from build123d import *

# Parameters (mm, degrees)
SKETCH1_W                      = 114.3
SKETCH1_H                      = 63.5
BASE_FLANGE1_DEPTH             = 2.032
EDGE_FLANGE1_STRIP_W           = 14.478
EDGE_FLANGE1_STRIP_H           = 2.032
EDGE_FLANGE1_STRIP_CUT_DEPTH   = 114.3
EDGE_FLANGE1_STRIP_2_W         = 14.478
EDGE_FLANGE1_STRIP_2_H         = 2.032
EDGE_FLANGE1_STRIP_CUT_2_DEPTH = 114.3
EDGE_FLANGE1_DEPTH             = 114.3
EDGE_FLANGE1_BEND_DEPTH        = 114.3
EDGE_FLANGE2_DEPTH             = 63.5
EDGE_FLANGE2_2_DEPTH           = 5.207
EDGE_FLANGE2_START             = 58.293
EDGE_FLANGE2_3_DEPTH           = 5.207
EDGE_FLANGE2_START_2           = 5.207
EDGE_FLANGE2_4_DEPTH           = 53.086
SKETCH15_R                     = 2.45745
CUT_EXTRUDE1_DEPTH             = 135.089147674
FILLET1_R                      = 3.175


# Read off the part's stored shape, not the designer's step: Edge-Flange2
# Sheet-metal steps are written as plain solids
with BuildPart() as part:
    # Sketch1 → Base-Flange1 (new body)
    with BuildSketch(Plane(origin=(0, 0, 0), x_dir=(0, 0, -1), z_dir=(1, 0, 0))):
        with Locations((57.15, 31.75)):
            Rectangle(SKETCH1_W, SKETCH1_H)
    extrude(amount=-BASE_FLANGE1_DEPTH)

    # Edge-Flange1 strip (across the edge) → Edge-Flange1 strip cut (cut)
    with BuildSketch(Plane(origin=(0, 63.5, -114.3), x_dir=(0, -1, 0), z_dir=(0, 0, 1))):
        with Locations((-2.032, -1.016)):
            Rectangle(EDGE_FLANGE1_STRIP_W, EDGE_FLANGE1_STRIP_H)
    extrude(amount=EDGE_FLANGE1_STRIP_CUT_DEPTH, mode=Mode.SUBTRACT)

    # Edge-Flange1 strip 2 (across the edge) → Edge-Flange1 strip cut 2 (cut)
    with BuildSketch(Plane.YX):
        with Locations((-2.032, -1.016)):
            Rectangle(EDGE_FLANGE1_STRIP_2_W, EDGE_FLANGE1_STRIP_2_H)
    extrude(amount=EDGE_FLANGE1_STRIP_CUT_2_DEPTH, mode=Mode.SUBTRACT)

    # Edge-Flange1 section (across the edge) → Edge-Flange1 (add)
    with BuildSketch(Plane(origin=(0, 63.5, -114.3), x_dir=(0, -1, 0), z_dir=(0, 0, 1))):
        with BuildLine():
            Line((0, 3.175), (0, 29.718))
            Line((0, 29.718), (2.032, 29.718))
            Line((2.032, 29.718), (2.032, 3.175))
            ThreePointArc((2.032, 3.175), (2.96193597, 0.92993597), (5.207, 0))
            Line((5.207, 0), (5.207, -2.032))
            ThreePointArc((5.207, -2.032), (1.52509499, -0.50690501), (0, 3.175))
        make_face()
    extrude(amount=EDGE_FLANGE1_DEPTH)

    # Edge-Flange1 section 2 (across the edge) → Edge-Flange1 bend (add)
    with BuildSketch(Plane.YX):
        with BuildLine():
            Line((0, 3.175), (0, 29.718))
            Line((0, 29.718), (2.032, 29.718))
            Line((2.032, 29.718), (2.032, 3.175))
            ThreePointArc((2.032, 3.175), (2.96193597, 0.92993597), (5.207, 0))
            Line((5.207, 0), (5.207, -2.032))
            ThreePointArc((5.207, -2.032), (1.52509499, -0.50690501), (0, 3.175))
        make_face()
    extrude(amount=EDGE_FLANGE1_BEND_DEPTH)

    # Edge-Flange2 outline → Edge-Flange2 (cut)
    with BuildSketch(Plane(origin=(0, 0, 0), x_dir=(1, 0, 0), z_dir=(0, 1, 0))):
        with BuildLine():
            Line((3.175, 0), (3.175, 3.175))
            Line((3.175, 3.175), (0, 3.175))
            ThreePointArc((0, 3.175), (0.92993597, 0.92993597), (3.175, 0))
        make_face()
        with BuildLine():
            ThreePointArc((-0.95201151, 0), (-1.754614485, 1.498172628), (-2.032, 3.175))
            Line((-2.032, 3.175), (-2.032, 0))
            Line((-2.032, 0), (-0.95201151, 0))
        make_face()
    extrude(amount=EDGE_FLANGE2_DEPTH, mode=Mode.SUBTRACT)

    # Edge-Flange2 2 outline → Edge-Flange2 2 (cut)
    with BuildSketch(Plane(origin=(0, 0, 0), x_dir=(1, 0, 0), z_dir=(0, 1, 0))):
        with BuildLine():
            ThreePointArc((3.175, 0), (0.92993597, 0.92993597), (0, 3.175))
            Line((0, 3.175), (-2.032, 3.175))
            ThreePointArc((-2.032, 3.175), (-1.754614485, 1.498172628), (-0.95201151, 0))
            Line((-0.95201151, 0), (3.175, 0))
        make_face()
    extrude(amount=EDGE_FLANGE2_2_DEPTH, mode=Mode.SUBTRACT)

    # Edge-Flange2 3 outline → Edge-Flange2 3 (cut)
    with BuildSketch(Plane(origin=(0, 0, 0), x_dir=(1, 0, 0), z_dir=(0, 1, 0)).offset(EDGE_FLANGE2_START)):
        with BuildLine():
            ThreePointArc((3.175, 0), (0.92993597, 0.92993597), (0, 3.175))
            Line((0, 3.175), (-2.032, 3.175))
            ThreePointArc((-2.032, 3.175), (-1.754614485, 1.498172628), (-0.95201151, 0))
            Line((-0.95201151, 0), (3.175, 0))
        make_face()
    extrude(amount=EDGE_FLANGE2_3_DEPTH, mode=Mode.SUBTRACT)

    # Edge-Flange2 4 outline → Edge-Flange2 4 (add)
    with BuildSketch(Plane(origin=(0, 0, 0), x_dir=(1, 0, 0), z_dir=(0, 1, 0)).offset(EDGE_FLANGE2_START_2)):
        with BuildLine():
            Line((0, 3.175), (0, 0))
            Line((0, 0), (-0.95201151, 0))
            ThreePointArc((-0.95201151, 0), (0.874932175, -1.496459836), (3.175, -2.032))
            Line((3.175, -2.032), (29.718, -2.032))
            Line((29.718, -2.032), (29.718, 0))
            Line((29.718, 0), (3.175, 0))
            ThreePointArc((3.175, 0), (0.92993597, 0.92993597), (0, 3.175))
        make_face()
    extrude(amount=EDGE_FLANGE2_4_DEPTH)

    # Sketch15 → Cut-Extrude1 (cut, through all)
    with BuildSketch(Plane(origin=(0, 63.5, 0), x_dir=(1, 0, 0), z_dir=(0, 1, 0))):
        with Locations(Location((17.018, 101.6, 0), (0, 0, 180))):
            Circle(SKETCH15_R)
        with Locations(Location((17.018, 12.7, 0), (0, 0, 180))):
            Circle(SKETCH15_R)
    extrude(amount=-CUT_EXTRUDE1_DEPTH, mode=Mode.SUBTRACT)

    # Fillet1
    fillet1_edges = [part.edges().sort_by_distance(p)[0] for p in [
        (29.718, 1.016, -114.3),
        (29.718, 62.484, -114.3),
        (3.175, 1.016, 0),
        (29.718, 1.016, 0),
        (29.718, 5.207, 1.016),
        (29.718, 58.293, 1.016),
        (29.718, 62.484, 0),
        (3.175, 62.484, 0),
    ]]
    fillet(fillet1_edges, radius=FILLET1_R - 0.0001)  # a hair under: the kernel refuses the full size


solid = part.part
Design review of the part built by this model. Coordinates are the model's own, in mm. A direction names the side the tool comes from. Give positions to 0.01 mm unless a question says otherwise; leave off trailing zeros. Write each loop counter-clockwise with the first axis right and the second up, starting at its lowest first coordinate (ties: lowest second). Pieces come first, ordered by that corner, then holes. Notation, with made-up numbers: M 8,28.5 L 34,28.5 A10 ccw 34,47.5 Z; hole C 1.25,30.25 d11. An arc over 180 degrees is marked long. Return JSON: item names as keys, results as strings. Group by question number.
Item 1: Take a section at A-A (z = -101.6). Give the boundary of the cut face in (x, y) (3 decimals).
Item 2: Tool access review of faces 4 (the flat face through (12, 5.207, 1)), 5 (the cylindrical face through (15.697, 62.498, -99.528)), 6 (the flat face through (17, 2.032, -56)), 7 (the cylindrical face through (28.76, 57.39, 1)), 8 (the flat face through (12, 58.293, 1)): name each direction out of +Z, -Z, +X, -X, +Y, -Y from which nothing blocks a thin tool from reaching the whole face with its end or side.
Item 3: The part is to be moulded in two halves that separate along X. For faces 1 (the cylindrical face through (28.763, 62.47, -113.395)), 2 (the cylindrical face through (15.88, 1.03, -14.88)), 3 (the flat face through (-0.4, 31.9, -114.3)), say which applies: pulls with the +X half, pulls with the -X half, needs draft (parallel to the pull), parting line crosses it, or undercut.
Item 4: Clearance check with flat-ended pins moving along their axes: pin 1 Ø4 at (y, z) = (46, -58.5) entering from +X; pin 2 Ø1.6 at (x, y) = (0.5, 62) entering from +Z (3 decimals); pin 3 Ø6 at (x, y) = (6, 11.5) entering from -Z; pin 4 Ø3 at (x, z) = (17.018, -12.7) entering from -Y. State where each tip first meets the part, or that it passes through.
Item 5: Take a section at D-D (z = -4.5). Give the boundary of the cut face in (x, y) (3 decimals), plus the area to 3 significant figures.
Item 6: Take a section at B-B (x = 24). Give the boundary of the cut face in (y, z).
Item 7: Wall thickness on line 1 along Y through (x, z) = (8.5, -20); line 2 along X through (y, z) = (10, -64); line 3 along Z through (x, y) = (7.5, 10): over which ranges is each line inside the solid? List them lowest first.
Item 8: Take a section at C-C (x = 18). Give the boundary of the cut face in (y, z).
Return value:
{
 "1": {"outline": "M -2.032,5.207 A5.207 ccw 3.175,0 L 14.561,0 L 14.561,2.032 L 3.175,2.032 A3.175 cw 0,5.207 L 0,58.293 A3.175 cw 3.175,61.468 L 14.561,61.468 L 14.561,63.5 L 3.175,63.5 A5.207 ccw -2.032,58.293 Z; M 19.475,0 L 29.718,0 L 29.718,2.032 L 19.475,2.032 Z; M 19.475,61.468 L 29.718,61.468 L 29.718,63.5 L 19.475,63.5 Z"},
 "2": {"face 4": "+Z, +X, -X, -Y", "face 5": "+Y, -Y", "face 6": "+Z, -Z, +X", "face 7": "+Z, -Z, +X, +Y", "face 8": "+Z, +X, -X, +Y"},
 "3": {"face 1": "pulls with the +X half", "face 2": "undercut", "face 3": "needs draft"},
 "4": {"pin 1": "stops at x = 0", "pin 2": "stops at z = -3.175", "pin 3": "stops at z = 0", "pin 4": "passes through"},
 "5": {"outline": "M -2.032,5.207 A5.207 ccw 3.175,0 L 29.718,0 L 29.718,2.032 L 3.175,2.032 A3.175 cw 0,5.207 L 0,58.293 A3.175 cw 3.175,61.468 L 29.718,61.468 L 29.718,63.5 L 3.175,63.5 A5.207 ccw -2.032,58.293 Z", "area": "242 mm2"},
 "6": {"outline": "M 0,-114.3 L 2.03,-114.3 L 2.03,0 L 0,0 Z; M 5.21,0 L 58.29,0 L 58.29,2.03 L 5.21,2.03 Z; M 61.47,-114.3 L 63.5,-114.3 L 63.5,0 L 61.47,0 Z"},
 "7": {"line 1": "y = 0 to 2.03, 61.47 to 63.5", "line 2": "x = -2.03 to 0", "line 3": "z = 0 to 2.03"},
 "8": {"outline": "M 0,-114.3 L 2.03,-114.3 L 2.03,-103.85 L 0,-103.85 Z; M 0,-99.35 L 2.03,-99.35 L 2.03,-14.95 L 0,-14.95 Z; M 0,-10.45 L 2.03,-10.45 L 2.03,0 L 0,0 Z; M 5.21,0 L 58.29,0 L 58.29,2.03 L 5.21,2.03 Z; M 61.47,-114.3 L 63.5,-114.3 L 63.5,-103.85 L 61.47,-103.85 Z; M 61.47,-99.35 L 63.5,-99.35 L 63.5,-14.95 L 61.47,-14.95 Z; M 61.47,-10.45 L 63.5,-10.45 L 63.5,0 L 61.47,0 Z"}
}
